```python
from build123d import *

# Parameters (mm, degrees)
F0_R     = 11.5
F0_R_2   = 1.75
F0_W     = 46.25
F0_H     = 25
F0_R_3   = 2.5
F1_DEPTH = 10
F2_R     = 5
F2_R_2   = 2.5
F3_DEPTH = 5


# Not quite as in the source:
# - a feature names something its author has since deleted; it is built from what else it names


with BuildPart() as f1:
    # F0 (on Top) → F1 (new body)
    with BuildSketch(Plane.XY):
        with BuildLine():
            Line((15.5000000202, 21.25), (-15.5, 21.25))
            ThreePointArc((-15.5, 21.25), (-11.4341360082, 19.5658639918), (-9.75, 15.5))
            ThreePointArc((-9.75, 15.5), (-15.5, 9.75), (-21.25, 15.5))
            Line((-21.25, 15.5), (-21.25, -15.4999999845))
            ThreePointArc((-21.25, -15.4999999845), (-15.4999999923, -9.75), (-9.75, -15.5))
            ThreePointArc((-9.75, -15.5), (-11.4341360082, -19.5658639918), (-15.5, -21.25))
            Line((-15.5, -21.25), (15.4999999923, -21.25))
            ThreePointArc((15.4999999923, -21.25), (11.4341360109, -11.4341360054), (21.25, -15.5))
            Line((21.25, -15.5), (21.25, -12.5))
            Line((21.25, -12.5), (21.25, 12.5))
            Line((21.25, 12.5), (21.25, 15.5))
            ThreePointArc((21.25, 15.5), (11.434136001, 11.4341360153), (15.5000000202, 21.25))
        make_face()
        Circle(F0_R, mode=Mode.SUBTRACT)
        with BuildLine():
            ThreePointArc((-9.75, -15.5), (-15.4999999923, -9.75), (-21.25, -15.4999999845))
            ThreePointArc((-21.25, -15.4999999845), (-19.5658639973, -19.5658639864), (-15.5, -21.25))
            ThreePointArc((-15.5, -21.25), (-11.4341360082, -19.5658639918), (-9.75, -15.5))
        make_face()
        with Locations((-15.5, -15.5)):
            Circle(F0_R_2, mode=Mode.SUBTRACT)
        with BuildLine():
            ThreePointArc((-9.75, 15.5), (-11.4341360082, 19.5658639918), (-15.5, 21.25))
            ThreePointArc((-15.5, 21.25), (-19.5658639918, 19.5658639918), (-21.25, 15.5))
            ThreePointArc((-21.25, 15.5), (-15.5, 9.75), (-9.75, 15.5))
        make_face()
        with Locations((-15.5, 15.5)):
            Circle(F0_R_2, mode=Mode.SUBTRACT)
        with BuildLine():
            ThreePointArc((21.25, 15.5), (19.565863999, 19.5658639847), (15.5000000202, 21.25))
            ThreePointArc((15.5000000202, 21.25), (11.434136001, 11.4341360153), (21.25, 15.5))
        make_face()
        with Locations((15.5, 15.5)):
            Circle(F0_R_2, mode=Mode.SUBTRACT)
        with BuildLine():
            ThreePointArc((21.25, -15.5), (11.4341360109, -11.4341360054), (15.4999999923, -21.25))
            ThreePointArc((15.4999999923, -21.25), (19.5658639891, -19.5658639946), (21.25, -15.5))
        make_face()
        with Locations((15.5, -15.5)):
            Circle(F0_R_2, mode=Mode.SUBTRACT)
        with Locations((44.375, 0)):
            Rectangle(F0_W, F0_H)
        with Locations((60, 0)):
            Circle(F0_R_3, mode=Mode.SUBTRACT)
    extrude(amount=F1_DEPTH)

    # F2 (on face) → F3 (cut)
    with BuildSketch(Plane.XY.offset(10)):
        with Locations((60, 0)):
            Circle(F2_R)
        with Locations((60, 0)):
            Circle(F2_R_2, mode=Mode.SUBTRACT)
    extrude(amount=-F3_DEPTH, mode=Mode.SUBTRACT)


solid = f1.part
```
Read the model definition and answer for the solid it produces. Units are mm, in the model's axes. A direction names the side the tool comes from. Coordinates: 2 decimals unless noted, no trailing zeros. Order: outer loops, then holes, each group sorted by start corner. A loop starts at its lowest first (then second) coordinate and runs counter-clockwise, first axis right, second up. Notation, with made-up numbers: (-10.5, 3) - (20.5, 3) arc R32 ccw to (20.5, 33) - close; hole circle Ø5 at (50, 84.25). An arc over 180 degrees is marked (long way). Answer as a JSON object with one key per item and string values. Group by question number.
Item 1: A tool of negligible diameter and unlimited length cuts with its end or side. For faces 4 (the face through (44, -12.5, 5)), 5 (the face through (44, 12.5, 5)), 6 (the face through (-14.6, 17, 4.9)), 7 (the face through (62, -2, 5)), from which of +Z, -Z, +X, -X, +Y, -Y can it reach the whole face along a straight path? Write none if from no direction.
Item 2: Flat-ended cylindrical pins translate along their axes: P1, Ø12, axis at x = -2.5, y = -3.5, coming from the +Z side; P2, Ø5, axis at x = 38, z = 5.5, coming from the -Y side; P3, Ø1.5, axis at x = 54, z = 3, coming from the +Y side; P4, Ø16, axis at x = 60, y = 0, coming from the +Z side. Find the tip coordinate at first contact, or state that the pin passes through.
Item 3: Section A-A (z = 7) is taken. Give the vertices of the cut face in (x, y), plus the area to 3 significant figures.
Item 4: The mould has two halves that part along X. Classify faces 1 (the face through (55, 0, 8)), 2 (the face through (-19.61, -19.52, 4.93)), 3 (the face through (19.52, -19.61, 4.93)): +X half, -X half, draft (parallel to the pull), parting line (faces both ways), or undercut.
Item 5: Section C-C (x = 1.5) is taken. Give the vertices of the cut face in (y, z).
Item 6: Section B-B (y = 0) is taken. Give the vertices of the cut face in (x, z).
Item 7: Consider probe 1 along X at (y, z) = (14, 2.5); probe 2 along Y at (x, z) = (-15.5, 4.5); probe 3 along Y at (x, z) = (42, 4.5). Determine where each line is inside the solid, lowest interval first. Write a range as from..to.
Item 8: Section D-D (y = 7) is taken. Give the vertices of the cut face in (x, z).
Results are:
{
 "1": {"face 4": "+Z, -Z, +X, -Y", "face 5": "+Z, -Z, +X, +Y", "face 6": "+Z, -Z", "face 7": "+Z"},
 "2": {"P1": "passes through", "P2": "stops at y = -12.5", "P3": "stops at y = 12.5", "P4": "stops at z = 10"},
 "3": {"outline": "(-21.25, -15.5) arc R5.75 ccw to (-15.5, -21.25) - (15.5, -21.25) arc R5.75 ccw to (21.25, -15.5) - (21.25, -12.5) - (67.5, -12.5) - (67.5, 12.5) - (21.25, 12.5) - (21.25, 15.5) arc R5.75 ccw to (15.5, 21.25) - (-15.5, 21.25) arc R5.75 ccw to (-21.25, 15.5) - close; hole circle Ø3.5 at (-15.5, -15.5); hole circle Ø3.5 at (-15.5, 15.5); hole circle Ø23 at (0, 0); hole circle Ø3.5 at (15.5, -15.5); hole circle Ø3.5 at (15.5, 15.5); hole circle Ø10 at (60, 0)", "area": "2,400 mm^2"},
 "4": {"face 1": "undercut", "face 2": "-X half", "face 3": "+X half"},
 "5": {"outline": "(-21.25, 0) - (-11.4, 0) - (-11.4, 10) - (-21.25, 10) - close; (11.4, 0) - (21.25, 0) - (21.25, 10) - (11.4, 10) - close"},
 "6": {"outline": "(-21.25, 0) - (-11.5, 0) - (-11.5, 10) - (-21.25, 10) - close; (11.5, 0) - (57.5, 0) - (57.5, 5) - (55, 5) - (55, 10) - (11.5, 10) - close; (62.5, 0) - (67.5, 0) - (67.5, 10) - (65, 10) - (65, 5) - (62.5, 5) - close"},
 "7": {"probe 1": "x = -21.25..-16.4, -14.6..14.6, 16.4..21.25", "probe 2": "y = -21.25..-17.25, -13.75..13.75, 17.25..21.25", "probe 3": "y = -12.5..12.5"},
 "8": {"outline": "(-21.25, 0) - (-9.12, 0) - (-9.12, 10) - (-21.25, 10) - close; (9.12, 0) - (67.5, 0) - (67.5, 10) - (9.12, 10) - close"}
}
